Model file for the job. Use its own axes, mm. Face numbers are marked on the shaded views. Coordinates: 2 decimals unless noted, no trailing zeros. Order: outer loops, then holes, each group sorted by start corner. A loop starts at its lowest first (then second) coordinate and runs counter-clockwise, first axis right, second up.
from build123d import *

# Parameters (mm, degrees)
SKETCH016_W                             = 90
SKETCH016_H                             = 2.6
PAD005_DEPTH                            = 65
POCKET006_DEPTH                         = 316.271517
POCKET006_DEPTH_BACK                    = 318.871517
POCKET006_LINEARPATTERN003_2_DEPTH      = 316.271517
POCKET006_LINEARPATTERN003_2_DEPTH_BACK = 318.871517
LINEARPATTERN004_COUNT                  = 4
LINEARPATTERN004_PITCH                  = 30
SKETCH018_W                             = 120
SKETCH018_H                             = 175
POCKET007_DEPTH                         = 2.601
PAD006_DEPTH                            = 30


with BuildPart() as part:
    # Sketch016 → Pad005 (new body, symmetric)
    with BuildSketch(Plane.XZ):
        with Locations((0, 1.3)):
            Rectangle(SKETCH016_W, SKETCH016_H)
    extrude(amount=PAD005_DEPTH, both=True)

    # Sketch017 → Pocket006 (cut, two sides)
    with BuildSketch(Plane.XY) as pocket006_sk:
        with BuildLine():
            ThreePointArc((-30, 57.87868), (-22.5, 55.300828), (-15, 57.87868))
            ThreePointArc((-15, 47.12132), (-13.270688, 52.5), (-15, 57.87868))
            ThreePointArc((-15, 47.12132), (-22.5, 49.699172), (-30, 47.12132))
            ThreePointArc((-30, 57.87868), (-31.729312, 52.5), (-30, 47.12132))
        make_face()
        with BuildLine():
            ThreePointArc((-2.12132, 60), (-7.5, 61.729312), (-12.87868, 60))
            ThreePointArc((-12.87868, 45), (-10.300828, 52.5), (-12.87868, 60))
            ThreePointArc((-12.87868, 45), (-7.5, 43.270688), (-2.12132, 45))
            ThreePointArc((-2.12132, 60), (-4.699172, 52.5), (-2.12132, 45))
        make_face()
        with BuildLine():
            ThreePointArc((-17.12132, 45), (-22.5, 46.729312), (-27.87868, 45))
            ThreePointArc((-27.87868, 30), (-25.300828, 37.5), (-27.87868, 45))
            ThreePointArc((-27.87868, 30), (-22.5, 28.270688), (-17.12132, 30))
            ThreePointArc((-17.12132, 45), (-19.699172, 37.5), (-17.12132, 30))
        make_face()
        with BuildLine():
            ThreePointArc((-15, 42.87868), (-16.729312, 37.5), (-15, 32.12132))
            ThreePointArc((0, 32.12132), (-7.5, 34.699172), (-15, 32.12132))
            ThreePointArc((0, 32.12132), (1.729312, 37.5), (0, 42.87868))
            ThreePointArc((-15, 42.87868), (-7.5, 40.300828), (0, 42.87868))
        make_face()
    pocket006 = extrude(amount=-POCKET006_DEPTH, mode=Mode.SUBTRACT) + extrude(pocket006_sk.sketch, amount=POCKET006_DEPTH_BACK, mode=Mode.SUBTRACT)

    # Sketch017 LinearPattern003 2 → Pocket006 LinearPattern003 2 (cut, two sides)
    with BuildSketch(Plane(origin=(30, 0, 0), x_dir=(1, 0, 0), z_dir=(0, 0, 1))) as pocket006_linearpattern003_2_sk:
        with BuildLine():
            ThreePointArc((-30, 57.87868), (-22.5, 55.300828), (-15, 57.87868))
            ThreePointArc((-15, 47.12132), (-13.270688, 52.5), (-15, 57.87868))
            ThreePointArc((-15, 47.12132), (-22.5, 49.699172), (-30, 47.12132))
            ThreePointArc((-30, 57.87868), (-31.729312, 52.5), (-30, 47.12132))
        make_face()
        with BuildLine():
            ThreePointArc((-2.12132, 60), (-7.5, 61.729312), (-12.87868, 60))
            ThreePointArc((-12.87868, 45), (-10.300828, 52.5), (-12.87868, 60))
            ThreePointArc((-12.87868, 45), (-7.5, 43.270688), (-2.12132, 45))
            ThreePointArc((-2.12132, 60), (-4.699172, 52.5), (-2.12132, 45))
        make_face()
        with BuildLine():
            ThreePointArc((-17.12132, 45), (-22.5, 46.729312), (-27.87868, 45))
            ThreePointArc((-27.87868, 30), (-25.300828, 37.5), (-27.87868, 45))
            ThreePointArc((-27.87868, 30), (-22.5, 28.270688), (-17.12132, 30))
            ThreePointArc((-17.12132, 45), (-19.699172, 37.5), (-17.12132, 30))
        make_face()
        with BuildLine():
            ThreePointArc((-15, 42.87868), (-16.729312, 37.5), (-15, 32.12132))
            ThreePointArc((0, 32.12132), (-7.5, 34.699172), (-15, 32.12132))
            ThreePointArc((0, 32.12132), (1.729312, 37.5), (0, 42.87868))
            ThreePointArc((-15, 42.87868), (-7.5, 40.300828), (0, 42.87868))
        make_face()
    pocket006_linearpattern003_2 = extrude(amount=-POCKET006_LINEARPATTERN003_2_DEPTH, mode=Mode.SUBTRACT) + extrude(pocket006_linearpattern003_2_sk.sketch, amount=POCKET006_LINEARPATTERN003_2_DEPTH_BACK, mode=Mode.SUBTRACT)

    # LinearPattern004: Pocket006, Pocket006 LinearPattern003 2 ×4
    with Locations(*[(0, -i * LINEARPATTERN004_PITCH, 0) for i in range(1, LINEARPATTERN004_COUNT)]):
        add(pocket006, mode=Mode.SUBTRACT)
        add(pocket006_linearpattern003_2, mode=Mode.SUBTRACT)

    # Sketch018 → Pocket007 (cut, through all)
    with BuildSketch(Plane.XY):
        Rectangle(SKETCH018_W, SKETCH018_H)
        with BuildLine():
            ThreePointArc((-30.150681, 59.846229), (-33.106055, 52.392354), (-30, 45))
            ThreePointArc((-30, 30), (-26.893398, 37.5), (-30, 45))
            ThreePointArc((-30, 30), (-33.106602, 22.5), (-30, 15))
            ThreePointArc((-30, 0), (-26.893398, 7.5), (-30, 15))
            ThreePointArc((-30, 0), (-33.106602, -7.5), (-30, -15))
            ThreePointArc((-30, -30), (-26.893398, -22.5), (-30, -15))
            ThreePointArc((-30, -30), (-33.106602, -37.5), (-30, -45))
            ThreePointArc((-29.849318, -59.846228), (-26.893945, -52.392354), (-30, -45))
            ThreePointArc((-29.849318, -59.846228), (-22.501092, -62.891321), (-15.152226, -59.847774))
            ThreePointArc((0.152226, -59.847774), (-7.5, -56.678118), (-15.152226, -59.847774))
            ThreePointArc((0.152226, -59.847774), (7.5, -62.891321), (14.847774, -59.847774))
            ThreePointArc((30.150681, -59.846229), (22.498908, -56.678118), (14.847774, -59.847774))
            ThreePointArc((30.150681, -59.846229), (33.106055, -52.392354), (30, -45))
            ThreePointArc((30, -30), (26.893398, -37.5), (30, -45))
            ThreePointArc((30, -30), (33.106602, -22.5), (30, -15))
            ThreePointArc((30, 0), (26.893398, -7.5), (30, -15))
            ThreePointArc((30, 0), (33.106602, 7.5), (30, 15))
            ThreePointArc((30, 30), (26.893398, 22.5), (30, 15))
            ThreePointArc((30, 30), (33.106602, 37.5), (30, 45))
            ThreePointArc((29.849318, 59.846228), (26.893945, 52.392354), (30, 45))
            ThreePointArc((29.849318, 59.846228), (22.501092, 62.891321), (15.152226, 59.847774))
            ThreePointArc((-0.152226, 59.847774), (7.5, 56.678118), (15.152226, 59.847774))
            ThreePointArc((-0.152226, 59.847774), (-7.5, 62.891321), (-14.847774, 59.847774))
            ThreePointArc((-30.150681, 59.846229), (-22.498908, 56.678118), (-14.847774, 59.847774))
        make_face(mode=Mode.SUBTRACT)
    extrude(amount=POCKET007_DEPTH, mode=Mode.SUBTRACT)

    # Sketch019 → Pad006 (join)
    with BuildSketch(Plane.XY):
        with BuildLine():
            ThreePointArc((-30.150681, 59.846229), (-33.106055, 52.392354), (-30, 45))
            ThreePointArc((-30, 30), (-26.893398, 37.5), (-30, 45))
            ThreePointArc((-30, 30), (-33.106602, 22.5), (-30, 15))
            ThreePointArc((-30, 0), (-26.893398, 7.5), (-30, 15))
            ThreePointArc((-30, 0), (-33.106602, -7.5), (-30, -15))
            ThreePointArc((-30, -30), (-26.893398, -22.5), (-30, -15))
            ThreePointArc((-30, -30), (-33.106602, -37.5), (-30, -45))
            ThreePointArc((-29.849318, -59.846228), (-26.893945, -52.392354), (-30, -45))
            ThreePointArc((-29.849318, -59.846228), (-22.501092, -62.891321), (-15.152226, -59.847774))
            ThreePointArc((0.152226, -59.847774), (-7.5, -56.678118), (-15.152226, -59.847774))
            ThreePointArc((0.152226, -59.847774), (7.5, -62.891321), (14.847774, -59.847774))
            ThreePointArc((30.150681, -59.846229), (22.498908, -56.678118), (14.847774, -59.847774))
            ThreePointArc((30.150681, -59.846229), (33.106055, -52.392354), (30, -45))
            ThreePointArc((30, -30), (26.893398, -37.5), (30, -45))
            ThreePointArc((30, -30), (33.106602, -22.5), (30, -15))
            ThreePointArc((30, 0), (26.893398, -7.5), (30, -15))
            ThreePointArc((30, 0), (33.106602, 7.5), (30, 15))
            ThreePointArc((30, 30), (26.893398, 22.5), (30, 15))
            ThreePointArc((30, 30), (33.106602, 37.5), (30, 45))
            ThreePointArc((29.849318, 59.846228), (26.893945, 52.392354), (30, 45))
            ThreePointArc((29.849318, 59.846228), (22.501092, 62.891321), (15.152226, 59.847774))
            ThreePointArc((-0.152226, 59.847774), (7.5, 56.678118), (15.152226, 59.847774))
            ThreePointArc((-0.152226, 59.847774), (-7.5, 62.891321), (-14.847774, 59.847774))
            ThreePointArc((-30.150681, 59.846229), (-22.498908, 56.678118), (-14.847774, 59.847774))
        make_face()
    extrude(amount=PAD006_DEPTH)


solid = part.part
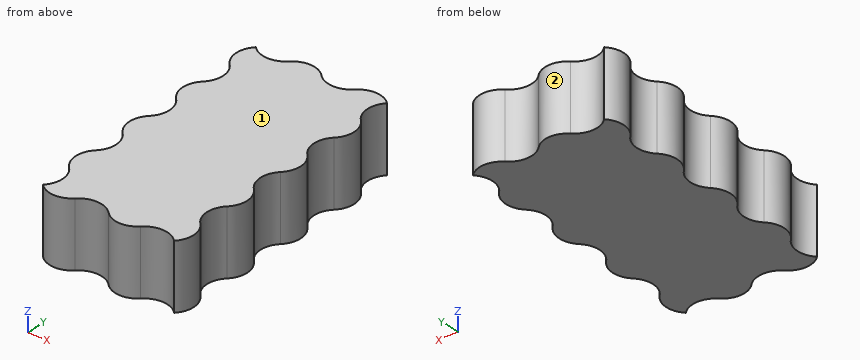
Q1. Probe line 1 (Y direction, x = 29.5, z = 8); line 2 (Y direction, x = -8, z = 8.5); line 3 (X direction, y = 31.5, z = 2). List the from-to ranges inside material, lowest first.
Established:
line 1: y = -59.25 to -44.46, -30.54 to -14.46, -0.54 to 15.54, 29.46 to 45.54, 59.46 to 60.18
line 2: y = -56.69 to 62.88
line 3: x = -28.75 to 31.25
Q2. Mould opens along X. For the marked faces 1 and 2 say: pulls with the +X half, pulls with the -X half, needs draft (parallel to the pull), parting line crosses it, or undercut.
Established:
face 1: needs draft
face 2: undercut
Q3. Drop flat-ended pins along their axis: P1, Ø3, axis at y = -18.5, z = 13.5, coming from the +X side; P2, Ø1.5, axis at x = -18, z = 26.5, coming from the +Y side; P3, Ø8, axis at y = 33, z = 19, coming from the +X side. Give the stop position or say it passes through.
Established:
P1: stops at x = 32.81
P2: stops at y = 58.04
P3: stops at x = 33.09
Q4. Cut at B-B, the plane x = -7. List the corners of the cut face in (y, z).
Established:
outline: (-56.69, 0) - (62.88, 0) - (62.88, 30) - (-56.69, 30) - close
Q5. Cut at C-C, the plane y = 50. List the corners of the cut face in (x, z), plus the area to 3 significant figures.
Established:
outline: (-32.81, 0) - (27.19, 0) - (27.19, 30) - (-32.81, 30) - close
area: 1,800 mm2
Q6. Cut at A-A, the plane z = 10.25. List the corners of the cut face in (x, y), plus the area to 3 significant figures.
Established:
outline: (-30.15, 59.85) arc R10.61 ccw to (-30, 45) arc R10.61 cw to (-30, 30) arc R10.61 ccw to (-30, 15) arc R10.61 cw to (-30, 0) arc R10.61 ccw to (-30, -15) arc R10.61 cw to (-30, -30) arc R10.61 ccw to (-30, -45) arc R10.61 cw to (-29.85, -59.85) arc R10.39 ccw to (-15.15, -59.85) arc R10.82 cw to (0.15, -59.85) arc R10.39 ccw to (14.85, -59.85) arc R10.82 cw to (30.15, -59.85) arc R10.61 ccw to (30, -45) arc R10.61 cw to (30, -30) arc R10.61 ccw to (30, -15) arc R10.61 cw to (30, 0) arc R10.61 ccw to (30, 15) arc R10.61 cw to (30, 30) arc R10.61 ccw to (30, 45) arc R10.61 cw to (29.85, 59.85) arc R10.39 ccw to (15.15, 59.85) arc R10.82 cw to (-0.15, 59.85) arc R10.39 ccw to (-14.85, 59.85) arc R10.82 cw to start
area: 7,170 mm2
